```python
from build123d import *

# Parameters (mm, degrees)
F1_DEPTH = 30
F2_W     = 24
F2_H     = 24
F2_R     = 5.1
F3_DEPTH = 3
F6_DEPTH = 4.5
F8_R     = 1


with BuildPart() as f1:
    # F0 (on Top) → F1 (new body)
    with BuildSketch(Plane.XY):
        with BuildLine():
            ThreePointArc((0, 13.5), (11.2743427126, 5.0323645735), (7.0706637066, -8.4264888743))
            ThreePointArc((7.0706637066, -8.4264888743), (7.1725693465, -10.2375673256), (8.8942921325, -10.8085844568))
            ThreePointArc((8.8942921325, -10.8085844568), (14.7842599605, 2.839809495), (6.2367777531, 15.0016731019))
            ThreePointArc((6.2367777531, 15.0016731019), (5.8102691618, 15.8862752393), (6.5779752006, 16.4986949957))
            Line((6.5779752006, 16.4986949957), (12, 16.4986949957))
            Line((12, 16.4986949957), (12, 19.4986949957))
            Line((12, 19.4986949957), (-12, 19.4986949957))
            Line((-12, 19.4986949957), (-12, 16.4986949957))
            Line((-12, 16.4986949957), (-6.5779752006, 16.4986949957))
            ThreePointArc((-6.5779752006, 16.4986949957), (-5.8102691618, 15.8862752393), (-6.2367777531, 15.0016731019))
            ThreePointArc((-6.2367777531, 15.0016731019), (-14.7842599605, 2.839809495), (-8.8942921325, -10.8085844568))
            ThreePointArc((-8.8942921325, -10.8085844568), (-7.1725693465, -10.2375673256), (-7.0706637066, -8.4264888743))
            ThreePointArc((-7.0706637066, -8.4264888743), (-11.2743427126, 5.0323645735), (0, 13.5))
        make_face()
    extrude(amount=F1_DEPTH)

    # F2 (on face) → F3 (join)
    with BuildSketch(Plane.XY.offset(30)):
        with Locations((0, 31.4986949957)):
            Rectangle(F2_W, F2_H)
        with Locations((0, 34.4986949957)):
            Circle(F2_R, mode=Mode.SUBTRACT)
    extrude(amount=-F3_DEPTH)

    # F4: union 

    # F5 (on face) → F6 (join)
    with BuildSketch(Plane.YZ.offset(12)):
        Polygon((19.4986949957, 27), (19.4986949957, 0), (43.4986949957, 27), align=None)
    extrude(amount=-F6_DEPTH)

    # F7: F1 across plane


with BuildPart() as f1_1:
    add(f1.part)
    add(f1.part.mirror(Plane.YZ))

    # F8
    f8_edges = [f1_1.edges().sort_by_distance(p)[0] for p in [
        (12, 17.998695, 0),
        (12, 16.498695, 15),
        (12, 29.998695, 30),
        (12, 43.498695, 28.5),
        (12, 31.498695, 13.5),
        (-12, 43.498695, 28.5),
        (-12, 29.998695, 30),
        (-12, 16.498695, 15),
        (-12, 17.998695, 0),
        (-12, 31.498695, 13.5),
    ]]
    fillet(f8_edges, radius=F8_R)


solid = f1_1.part
```
Geometry check sheet. Reference: the model listing, model coordinates, mm. A direction names the side the tool comes from. Coordinates: 2 decimals unless noted, no trailing zeros. Order: outer loops, then holes, each group sorted by start corner. A loop starts at its lowest first (then second) coordinate and runs counter-clockwise, first axis right, second up. Notation, with made-up numbers: M 49.25,65 L 58.25,65 A10 cw 58.25,70 Z; hole C -34.75,-10 d5. An arc over 180 degrees is marked long. One line per question, with ' | ' between items. Start each with the question number.
Item 1: Cross-section at C-C on y = 11.5. Enter the section's corners in (x, z).
Item 2: Cross-section at B-B on x = -1.5. Enter the section's corners in (y, z).
Item 3: Cross-section at A-A on y = -2. Enter the section's corners in (x, z), then the cut area to 3 significant figures.
Item 4: Draft check along Y on faces 1 (the flat face through (-12, 27, 18)), 2 (the cylindrical face through (11.21, 5.23, 14.79)), 3 (the flat face through (-9.27, 31.33, 13.31)). Enter one of: pulls with the +Y half, pulls with the -Y half, needs draft (parallel to the pull), parting line crosses it, or undercut.
Item 5: Set-up check for faces 4 (the cylindrical face through (-11.337, 4.832, 14.79)), 5 (the flat face through (-9, 16.499, 15)), 6 (the flat face through (9, 16.499, 15)), 7 (the flat face through (3.2, 13.4, 0)), 8 (the flat face through (7.5, 29, 17)): record each of +Z, -Z, +X, -X, +Y, -Y from which the full face is reachable in a straight line by a thin tool's end or side.
Item 6: Material ranges on L1, parallel to Y at x = 0, z = 28.6; L2, parallel to X at y = 25, z = 21.5; L3, parallel to Y at x = -10.25, z = 7, recorded low to high. Write a range as [from, to].
Item 7: Gauge pin test, flat ends, axial feed: pin 1 (12 mm diameter, centred on y = 26, z = 8.5, fed in from +X); pin 2 (8 mm diameter, centred on y = 0, z = 8.5, fed in from +X); pin 3 (4 mm diameter, centred on x = 2.5, y = 22.5, fed in from -Z); pin 4 (7.5 mm diameter, centred on y = 24, z = 17.5, fed in from -X). Record the tip position at first contact, or that the pin passes through.
Findings:
1) outline: M -10.92,0 L -6.35,0 L -6.35,30 L -10.92,30 Z; M 6.35,0 L 10.92,0 L 10.92,30 L 6.35,30 Z
2) outline: M 13.36,0 L 19.5,0 L 19.5,27 L 29.62,27 L 29.62,30 L 13.36,30 Z; M 39.37,27 L 43.5,27 L 43.5,30 L 39.37,30 Z
3) outline: M -14.51,0 L -11.42,0 L -11.42,30 L -14.51,30 Z; M 11.42,0 L 14.51,0 L 14.51,30 L 11.42,30 Z | area: 185 mm²
4) face 1: needs draft | face 2: undercut | face 3: pulls with the +Y half
5) face 4: +Z, -Z | face 5: +Z, -Z, -X | face 6: +Z, -Z, +X | face 7: -Z, +X, -X, +Y, -Y | face 8: -Z, +Y
6) L1: y = [13.5, 29.4], [39.6, 43.5] | L2: x = [-12, -7.5], [7.5, 12] | L3: y = [-9.64, -4.79], [7.35, 12.2], [16.5, 25.72]
7) pin 1: stops at x = 12 | pin 2: stops at x = 14.86 | pin 3: stops at z = 27 | pin 4: stops at x = -12
